For this review, take the finished solid that the model builds, in its own axes (mm). Give positions to 0.01 mm unless a question says otherwise; leave off trailing zeros. Loops run counter-clockwise (first coordinate to the right, second up) from the corner with the lowest first, then second, coordinate; pieces in that order, holes last. Notation, with made-up numbers: (59, 24.25) -> (93, 24.25) arc R17 ccw to (93, 53.25) -> close; hole circle Ø10 at (25, -1). An arc over 180 degrees is marked (long way). One line per question, with ' | ' between items. Start each with the question number.
(1) Wall thickness on probe 1 along Y at (x, z) = (-8, -2.6); probe 2 along X at (y, z) = (-6, -1.25); probe 3 along Y at (x, z) = (-8.75, -1.2): over which ranges is each line inside the solid? List them lowest first.
(2) Draft analysis for pull direction X (two halves, no side actions). For faces 1 (the cylindrical face through (-7.176, 6.345, -2.535)), 2 (the cylindrical face through (3.772, 3.004, -0.246)), state which applies: +X half, -X half, draft (parallel to the pull), parting line (faces both ways), or undercut.
(3) Insertion check: P1, Ø11.5, axis at x = -5.77, y = 0, coming from the -Z side; P2, Ø2, axis at x = -13, z = -2, coming from the -Y side; P3, Ø2, axis at x = -11, z = -2, coming from the +Y side. Each pin has a flat end and moves straight along its axis. Give the tip position at first contact, or say it passes through.
(4) Consider section A-A (z = -2.3). Write out the cut boundary in (x, y).
Autodesk Inventor part; units mm, degrees
ref_plane "YZ Plane" through (0, 0, 0) normal (1, 0, 0) x (0, 1, 0)
ref_plane "XZ Plane" through (0, 0, 0) normal (0, 1, 0) x (-1, 0, 0)
ref_plane "XY Plane" through (0, 0, 0) normal (0, 0, 1) x (1, 0, 0)
sketch "Skizze1" plane through (0, 0, 0) normal (0, 0, 1) x (1, 0, 0)
  circle A0 centre (-5.7665, 0) radius 6.5
  circle A1 centre (-5.7665, 0) radius 10
  point P0 (0, 0)
  dimension "d0" = 20
sketch "Skizze2" plane through (0, 0, 0) normal (1, 0, 0) x (0, 1, 0)
  line L0 (6.5, 0) -> (-6.5, 0) construction
  line L1 (10, 0) -> (-10, 0) construction
  line L2 (10, 0) -> (10, -0.5)
  arc A0 (10, -0.5) -> (8, -2.5) centre (10, -2.5) ccw
  line L3 (6.5, -4.8) -> (6.5, -0.2) construction
  line L4 (8, -2.5) -> (6.5, -2.5) construction
  line L5 (10, -5) -> (10, -4.5)
  arc A1 (8, -2.5) -> (10, -4.5) centre (10, -2.5) ccw
  line L6 (8, -2.5) -> (8, -1.525) construction
  line L7 (10, -0.5) -> (8.7772, -0.5) construction
  point P0 (0, 0)
  dimension "d4" = 1.5
ref_plane "Arbeitsebene1" through (-5.7665, 0, 0) normal (1, 0, 0) x (0, 1, 0)
sketch "Skizze3" plane through (-5.7665, 0, 0) normal (1, 0, 0) x (0, 1, 0)
  line L0 (10, 0) -> (10, -0.5)
  arc A0 (10, -0.5) -> (8, -2.5) centre (10, -2.5) ccw
  arc A1 (8, -2.5) -> (10, -4.5) centre (10, -2.5) ccw
  line L1 (10, -5) -> (10, -4.5)
  line L2 (10, -5) -> (6.5, -5)
  line L3 (6.5, -5) -> (6.5, 0)
  line L4 (6.5, 0) -> (10, 0)
  line L5 (6.5, -4.8) -> (6.5, -0.2)
  line L6 (6.3, -5) -> (-6.3, -5)
  point P0 (0, 0)
  dimension "d9" = 8
sweep "Sweeping2" add profiles "Skizze3" path "Skizze1" path curves A1
properties part number "Umlenkfläche" material "PC/ABS-Kunststoff, Umlenkrolle"
A:
1) probe 1: y = -7.68 to -6.1, 6.1 to 7.68 | probe 2: x = -11.7 to -8.27, -3.27 to 0.17 | probe 3: y = -7.94 to -5.77, 5.77 to 7.94
2) face 1: undercut | face 2: parting line
3) P1: passes through | P2: stops at y = -5.3 | P3: stops at y = 7.11
4) outline: circle Ø16.02 at (-5.77, 0); hole circle Ø13 at (-5.77, 0)
